Autodesk Inventor part; units mm, degrees
ref_plane "YZ Plane" through (0, 0, 0) normal (1, 0, 0) x (0, 1, 0)
ref_plane "XZ Plane" through (0, 0, 0) normal (0, 1, 0) x (-1, 0, 0)
ref_plane "XY Plane" through (0, 0, 0) normal (0, 0, 1) x (1, 0, 0)
sketch "Skizze1" plane through (0, 0, 0) normal (0, 1, 0) x (-1, 0, 0)
  line L0 (50.5762, -64.7123) -> (8.5762, -64.7123)
  line L1 (8.5762, -64.7123) -> (8.5762, -84.3623)
  line L2 (8.5762, -84.3623) -> (50.5762, -84.3623)
  line L3 (54.0762, -68.7123) -> (54.0762, -32.0373)
  line L4 (54.0762, -32.0373) -> (108.5762, -32.0373)
  line L5 (108.5762, -32.0373) -> (108.5762, -24.0373)
  line L6 (108.5762, -24.0373) -> (50.5762, -24.0373)
  line L7 (50.5762, -24.0373) -> (50.5762, -64.7123)
  line L8 (54.0762, -117.0373) -> (108.5762, -117.0373)
  line L9 (108.5762, -117.0373) -> (108.5762, -125.0373)
  line L10 (108.5762, -125.0373) -> (50.5762, -125.0373)
  line L11 (50.5762, -125.0373) -> (50.5762, -84.3623)
  line L12 (54.0762, -80.3623) -> (54.0762, -117.0373)
  line L13 (12.0762, -68.7123) -> (12.0762, -80.3623)
  line L14 (12.0762, -68.7123) -> (54.0762, -68.7123)
  line L15 (54.0762, -80.3623) -> (12.0762, -80.3623)
  point P0 (0, 0)
  dimension "d1" = 8
  dimension "d2" = 3.5
  dimension "d5" = 8
  dimension "d9" = 4
  dimension "d10" = 100
  dimension "d11" = 11.65
  dimension "d27" = 3.5
  dimension "d29" = 42
  dimension "d30" = 85
  dimension "d31" = 36.675
extrude "Extrusion1" add sketch "Skizze1" along normal blind 20
sketch "Skizze3" plane through (-12.0762, 0, -68.7123) normal (0, 0, -1) x (-1, 0, 0)
  line L0 (39, 0) -> (23.696, 15.304)
  line L1 (37.5, 0) -> (22.946, 14.554)
  line L2 (22.946, 14.554) -> (23.696, 15.304)
  line L3 (42, 0) -> (42, 20)
  line L4 (42, -13) -> (42, 0)
  line L5 (37.5, 0) -> (39, 0)
  line L6 (0, 0) -> (42, 0)
  point P0 (-12.0762, 0)
  point P1 (-3.5, 0)
  dimension "d19" = 1.5
  dimension "d21" = 15.304
  dimension "d26" = 41
extrude "Extrusion3" cut sketch "Skizze3" against normal blind 2.5
sketch "Skizze4" plane through (-108.5762, 0, -24.0373) normal (0, 0, 1) x (1, 0, 0)
  line L0 (0, 0) -> (0, 20)
  circle A0 centre (0, 10) radius 5
  point P0 (108.5762, 0)
  dimension "d32" = 10
extrude "Extrusion4" cut sketch "Skizze4" against normal blind 200
sketch "Skizze5" plane through (-54.0762, 0, -80.3623) normal (0, 0, 1) x (1, 0, 0)
  point P0 (54.0762, 0)
sketch "Skizze6" plane through (-54.0762, 0, -80.3623) normal (0, 0, 1) x (1, 0, 0)
  line L0 (0, 0) -> (42, 0)
  line L1 (4.5, 0) -> (19.804, 15.304)
  line L2 (19.804, 15.304) -> (19.8768, 16.8022)
  line L3 (19.8768, 16.8022) -> (3, 0)
  line L4 (0, 0) -> (0, -2.9867)
  line L5 (4.5, 0) -> (0, 0)
  point P0 (54.0762, 0)
  point P1 (45.5, 0)
  dimension "d35" = 45
  dimension "d36" = 15.304
  dimension "d37" = 1.5
  dimension "d38" = 1.5
  dimension "d39" = 41
extrude "Extrusion5" cut sketch "Skizze6" against normal blind 2.5
sketch "Skizze7" plane through (-108.5762, 20, -32.0373) normal (-1, 0, 0) x (0, 0, 1)
  line L0 (8, -5) -> (8, 0)
  line L1 (8, -15) -> (0, -15)
  line L2 (0, -5) -> (8, -5)
  line L3 (-93, -5) -> (-93, 0)
  point P0 (32.0373, -20)
  point P1 (4, -2.5)
  point P2 (3.7984, -17.5)
  point P3 (-89, -2.5)
  point P4 (-89, -17.5)
  dimension "d42" = 4
  dimension "d43" = 2.5
  dimension "d44" = 2.5
  dimension "d52" = 4
hole "Bohrung1" at (-108.5762, 17.5, -28.0373) at (-108.5762, 2.5, -28.2389) direction (1, 0, 0) diameter 2.75 depth 8 tip angle 118
sketch "Skizze8" plane through (-108.5762, 0, -125.0373) normal (-1, 0, 0) x (0, 0, 1)
  line L0 (8, 15) -> (8, 20)
  line L1 (0, 20) -> (8, 20)
  line L2 (0, 0) -> (8, 0)
  point P0 (125.0373, 0)
  point P1 (4, 17.5)
  point P2 (3.9503, 2.5)
  dimension "d53" = 4
  dimension "d54" = 2.5
  dimension "d55" = 2.5
hole "Bohrung2" at (-108.5762, 2.5, -121.087) at (-108.5762, 17.5, -121.0373) direction (1, 0, 0) diameter 2.75 depth 8 tip angle 118
sketch "Skizze9" plane through (-8.5762, 0, -64.7123) normal (1, 0, 0) x (0, 0, -1)
  line L0 (0, 0) -> (0, 20)
  line L1 (0, 0) -> (19.65, 0)
  point P0 (-64.7123, 0)
  point P1 (10, 10)
  dimension "d63" = 10
  dimension "d64" = 10
hole "Bohrung3" at (-8.5762, 10, -74.7123) direction (-1, 0, 0) diameter 10 depth 5 tip angle 118
sketch "Skizze12" plane through (-108.5762, 0, -24.0373) normal (0, 0, 1) x (1, 0, 0)
  line L0 (58, 20) -> (0, 20)
  line L1 (0, 0) -> (25, 0)
  line L2 (25, 0) -> (25, 20)
  line L3 (25, 20) -> (0, 20)
  line L4 (0, 20) -> (0, 0)
  point P0 (108.5762, 0)
  dimension "d75" = 25
  dimension "d76" = 20
extrude "Extrusion6" cut sketch "Skizze12" against normal blind 120
sketch "Skizze13" plane through (-50.5762, 0, -24.0373) normal (0, 0, 1) x (1, 0, 0)
  line L0 (-33, 0) -> (-33, 20)
  circle A0 centre (-33, 10) radius 5
  point P0 (50.5762, 0)
  dimension "d79" = 10
extrude "Extrusion7" cut sketch "Skizze13" against normal blind 120
sketch "Skizze14" plane through (-83.5762, 0, -32.0373) normal (-1, 0, 0) x (0, 0, 1)
  line L0 (8, 5) -> (0, 5)
  line L1 (0, 0) -> (0, 5)
  line L2 (0, 20) -> (8, 20)
  line L3 (8, 20) -> (8, 15)
  line L4 (-85, 5) -> (-93, 5)
  line L5 (-85, 5) -> (-85, 0)
  line L6 (-93, 20) -> (-85, 20)
  line L7 (-85, 20) -> (-85, 15)
  point P0 (32.0373, 0)
  point P1 (4, 2.5)
  point P2 (4, 17.5)
  point P3 (-89, 2.5)
  point P4 (-89, 17.5)
  dimension "d82" = 2.5
  dimension "d83" = 4
  dimension "d84" = 2.5
  dimension "d85" = 4
  dimension "d86" = 2.5
  dimension "d87" = 4
  dimension "d88" = 2.5
  dimension "d89" = 4
hole "Bohrung4" at (-83.5762, 2.5, -28.0373) at (-83.5762, 17.5, -28.0373) at (-83.5762, 17.5, -121.0373) at (-83.5762, 2.5, -121.0373) direction (1, 0, 0) diameter 3 depth 8 tip angle 118
ref_plane "Arbeitsebene3" through (-43.5762, 0, -64.7123) normal (1, 0, 0) x (0, 0, -1)
ref_plane "Arbeitsebene4" through (-83.5762, 17.5, -24.0373) normal (-1, 0, 0) x (0, 0, 1)
sketch "Skizze15" plane through (-83.5762, 17.5, -24.0373) normal (-1, 0, 0) x (0, 0, 1)
  point P0 (24.0373, -17.5)
  point P1 (-50.5568, -7.548)
sketch "Skizze16" plane through (-43.5762, 0, -64.7123) normal (1, 0, 0) x (0, 0, -1)
  point P0 (-64.7123, 0)
  point P1 (9.9474, 9.9802)
properties part number "Neue Grundplatte"
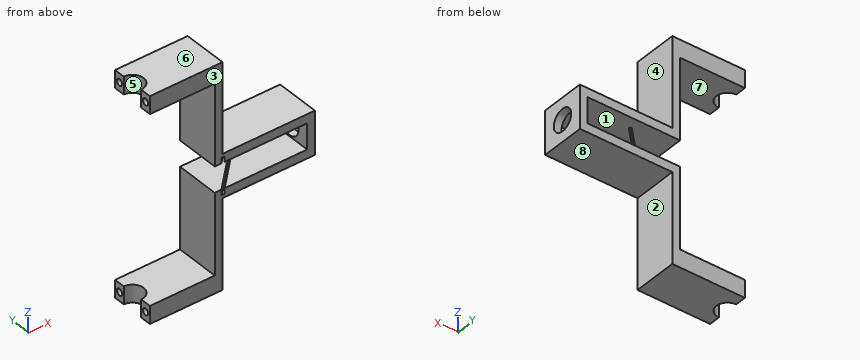
CAD build for the part. Positions are in the model's coordinates, mm. Face numbers are marked on the shaded views. A direction names the side the tool comes from. Round coordinates to 2 decimals unless told otherwise and drop trailing zeros. Order: outer loops, then holes, each group sorted by start corner. A loop starts at its lowest first (then second) coordinate and runs counter-clockwise, first axis right, second up. Notation, with made-up numbers: (44, 5.5) - (98, 5.5) arc R15 ccw to (98, 33.5) - close; hole circle Ø4 at (7.5, 3). An arc over 180 degrees is marked (long way). Answer as CSV lines item,"result". Start each with the question number.
1. Saw through at C-C, the plane z = -58.5. Write the cut outline in (x, y), and give its area (3 significant figures).
2. Saw through at D-D, the plane y = 6.5. Write the cut outline in (x, z).
3. Pull direction Z, two halves, no side cores. Call the marked faces 5, 6, 7 and 8: +Z half, -Z half, draft (parallel to the pull), parting line (faces both ways), or undercut.
4. Drill centre lines: L1, parallel to Z at x = -81, y = 2.5; L2, parallel to Z at x = -26.5, y = 9.5; L3, parallel to X at y = 12.75, z = -60.5. Where is each one in solid material? Low to high. Write a range as [from, to].
5. Saw through at A-A, the plane y = 12. Write the cut outline in (x, z), and give its area (3 significant figures).
6. Pin check, flat tips, straight feed: pin 1 (6 mm diameter, centred on y = 11.5, z = -101.5, fed in from +X); pin 2 (4 mm diameter, centred on y = 3.5, z = -98, fed in from -X); pin 3 (1.8 mm diameter, centred on y = 2.5, z = -121.04, fed in from -X). Stop position of each tip, or through.
7. Tool access for the marked faces 1, 2, 3 and 4: list every direction of +Z, -Z, +X, -X, +Y, -Y with a clear straight run to the whole face (end or side of a thin tool).
8. Saw through at B-B, the plane z = -77.5. Write the cut outline in (x, y), and give its area (3 significant figures).
Model answer:
1,outline,"(-54.08, 0) - (-50.58, 0) - (-50.58, 20) - (-54.08, 20) - close"
1,area,"70.0 mm²"
2,outline,"(-80.01, -125.04) - (-50.58, -125.04) - (-50.58, -84.36) - (-8.58, -84.36) - (-8.58, -78.28) - (-12.08, -78.28) - (-12.08, -80.36) - (-43.08, -80.36) - (-43.08, -82.86) - (-44.55, -82.86) - (-44.55, -80.36) - (-54.08, -80.36) - (-54.08, -117.04) - (-80.01, -117.04) - close; (-80.01, -32.04) - (-54.08, -32.04) - (-54.08, -68.71) - (-44.58, -68.71) - (-44.58, -66.21) - (-43.08, -66.21) - (-43.08, -68.71) - (-12.08, -68.71) - (-12.08, -71.14) - (-8.58, -71.14) - (-8.58, -64.71) - (-50.58, -64.71) - (-50.58, -24.04) - (-80.01, -24.04) - close"
3,face 5,"draft"
3,face 6,"+Z half"
3,face 7,"undercut"
3,face 8,"-Z half"
4,L1,"z = [-125.04, -122.54], [-119.54, -117.04], [-32.04, -29.54], [-26.54, -24.04]"
4,L2,"z = [-84.36, -80.36], [-68.71, -64.71]"
4,L3,"x = [-54.08, -50.58]"
5,outline,"(-78.99, -125.04) - (-50.58, -125.04) - (-50.58, -84.36) - (-8.58, -84.36) - (-8.58, -79.29) - (-12.08, -79.29) - (-12.08, -80.36) - (-37.58, -80.36) - (-37.58, -82.86) - (-39.02, -82.86) - (-39.02, -80.36) - (-54.08, -80.36) - (-54.08, -117.04) - (-78.99, -117.04) - close; (-78.99, -32.04) - (-54.08, -32.04) - (-54.08, -68.71) - (-39.08, -68.71) - (-39.08, -66.21) - (-37.58, -66.21) - (-37.58, -68.71) - (-12.08, -68.71) - (-12.08, -70.13) - (-8.58, -70.13) - (-8.58, -64.71) - (-50.58, -64.71) - (-50.58, -24.04) - (-78.99, -24.04) - close"
5,area,"1,050 mm²"
6,pin 1,"stops at x = -50.58"
6,pin 2,"stops at x = -54.08"
6,pin 3,"stops at x = -75.22"
7,face 1,"-X, +Y, -Y"
7,face 2,"-Z, +X, +Y, -Y"
7,face 3,"+Z, -Z, +X, -X, -Y"
7,face 4,"+Z, +X, +Y, -Y"
8,outline,"(-12.08, 0) - (-8.58, 0) - (-8.58, 5.85) - (-12.08, 5.85) - close; (-12.08, 14.15) - (-8.58, 14.15) - (-8.58, 20) - (-12.08, 20) - close"
8,area,"40.9 mm²"
